from build123d import *

# Parameters (mm, degrees)
F0_W     = 152
F0_H     = 38
F1_DEPTH = 3
F3_DEPTH = 1.5
F4_R     = 2


with BuildPart() as f1:
    # F0 (on Front) → F1 (new body)
    with BuildSketch(Plane.XZ):
        Rectangle(F0_W, F0_H)
    extrude(amount=F1_DEPTH)

    # F2 (on face) → F3 (cut)
    with BuildSketch(Plane.XZ.offset(3)):
        Polygon((-72.2, 19), (-76, 19), (-76, -19), (76, -19), (76, 19), (72.2, 19), (72.2, -15.2), (-72.2, -15.2), align=None)
    extrude(amount=-F3_DEPTH, mode=Mode.SUBTRACT)

    # F4
    f4_edges = [f1.edges().sort_by_distance(p)[0] for p in [
        (76, -0.75, -19),
        (72.2, -2.25, -15.2),
        (-76, -0.75, -19),
        (-72.2, -2.25, -15.2),
    ]]
    fillet(f4_edges, radius=F4_R)


solid = f1.part
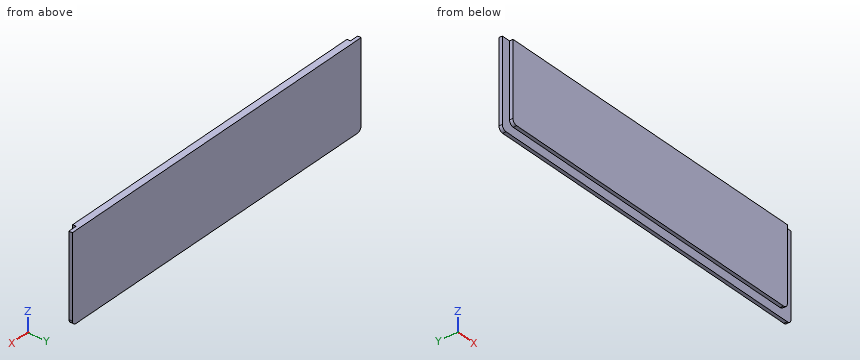
Here's how the part is built. I have some questions about the finished solid (model axes, mm). Coordinates: 2 decimals unless noted, no trailing zeros. Loops run counter-clockwise (first coordinate to the right, second up) from the corner with the lowest first, then second, coordinate; pieces in that order, holes last.
1. For P1, Ø1.6, axis at x = 29, y = -2.5, coming from the -Z side; P2, Ø1.5, axis at x = -9, z = -6.5, coming from the +Y side; P3, Ø0.8, axis at y = -2.5, z = 9.5, coming from the -X side, each with a flat end and sliding along its axis, tell me the tip position at first contact or that it passes through.
2. I need wall thicknesses on L1, parallel to X at y = -1.55, z = 11; L2, parallel to Y at x = -61, z = -16; L3, parallel to Z at x = 19, y = -2.3. Which ranges of each line are inside material? Lowest first, please.
3. Imagine slicing it at A-A, the plane z = -3.5. Please give me the cut outline in (x, y).
4. Imagine slicing it at B-B, the plane x = -49.5. Please give me the cut outline in (y, z), and give its area (3 significant figures).
Taken from the geometry:
1. P1: stops at z = -15.2
1. P2: stops at y = 0
1. P3: stops at x = -72.2
2. L1: x = -72.2 to 72.2
2. L2: y = -1.5 to 0
2. L3: z = -15.2 to 19
3. outline: (-76, -1.5) - (-72.2, -1.5) - (-72.2, -3) - (72.2, -3) - (72.2, -1.5) - (76, -1.5) - (76, 0) - (-76, 0) - close
4. outline: (-3, -15.2) - (-1.5, -15.2) - (-1.5, -19) - (0, -19) - (0, 19) - (-3, 19) - close
4. area: 108 mm2
